```python
from build123d import *

# Parameters (mm, degrees)
SKETCH1_R               = 12.7
BOSS_EXTRUDE1_DEPTH     = 1
CUT_EXTRUDE1_DEPTH      = 18.98832955
CUT_EXTRUDE1_DEPTH_BACK = 18.98832955
SKETCH19_R              = 1
CUT_EXTRUDE2_DEPTH      = 18.98832955
CUT_EXTRUDE2_DEPTH_BACK = 18.98832955
SKETCH20_R              = 7.5
SKETCH21_W              = 65.874202484
SKETCH21_H              = 51.979273979
CUT_EXTRUDE3_DEPTH      = 18.98832955
CUT_EXTRUDE4_DEPTH      = 18.98832955
CUT_EXTRUDE4_DEPTH_BACK = 18.98832955
SKETCH22_R              = 1
SKETCH22_R_2            = 0.25


with BuildPart() as part:
    # Sketch1 → Boss-Extrude1 (new body)
    with BuildSketch(Plane(origin=(0, 0, 0), x_dir=(1, 0, 0), z_dir=(0, 1, 0))):
        with Locations(Location((0, 0, 0), (0, 0, 270))):
            Circle(SKETCH1_R)
    extrude(amount=BOSS_EXTRUDE1_DEPTH)

    # Sketch19 → Cut-Extrude1 (cut, two sides: drawn at the far end of the back side and taken through both)
    with BuildSketch(Plane(origin=(0, 1, 0), x_dir=(1, 0, 0), z_dir=(0, 1, 0)).offset(-CUT_EXTRUDE1_DEPTH_BACK)):
        with Locations(Location((0, 11, 0), (0, 0, 270))):
            Circle(SKETCH19_R)
        with Locations(Location((9.526279442, 5.5, 0), (0, 0, 270))):
            Circle(SKETCH19_R)
        with Locations(Location((9.526279442, -5.5, 0), (0, 0, 270))):
            Circle(SKETCH19_R)
        with Locations(Location((0, -11, 0), (0, 0, 270))):
            Circle(SKETCH19_R)
        with Locations(Location((-9.526279442, -5.5, 0), (0, 0, 270))):
            Circle(SKETCH19_R)
        with Locations(Location((-9.526279442, 5.5, 0), (0, 0, 270))):
            Circle(SKETCH19_R)
    extrude(amount=CUT_EXTRUDE1_DEPTH + CUT_EXTRUDE1_DEPTH_BACK, mode=Mode.SUBTRACT)

    # Sketch20 → Cut-Extrude2 (cut, two sides: drawn at the far end of the back side and taken through both)
    with BuildSketch(Plane(origin=(0, 1, 0), x_dir=(1, 0, 0), z_dir=(0, 1, 0)).offset(-CUT_EXTRUDE2_DEPTH_BACK)):
        with Locations(Location((0, 0, 0), (0, 0, 270))):
            Circle(SKETCH20_R)
    extrude(amount=CUT_EXTRUDE2_DEPTH + CUT_EXTRUDE2_DEPTH_BACK, mode=Mode.SUBTRACT)

    # Sketch21 → Cut-Extrude3 (cut, through all)
    with BuildSketch(Plane.XY):
        with Locations((-3.816154381, 6.321647006)):
            Rectangle(SKETCH21_W, SKETCH21_H)
    extrude(amount=CUT_EXTRUDE3_DEPTH, mode=Mode.SUBTRACT)

    # Sketch22 → Cut-Extrude4 (cut, two sides: drawn at the far end of the back side and taken through both)
    with BuildSketch(Plane(origin=(0, 1, 0), x_dir=(1, 0, 0), z_dir=(0, 1, 0)).offset(-CUT_EXTRUDE4_DEPTH_BACK)):
        with Locations(Location((2.847009496, 10.625184089, 0), (0, 0, 270))):
            Circle(SKETCH22_R)
        with Locations(Location((-5.125, 8.876760389, 0), (0, 0, 270))):
            Circle(SKETCH22_R_2)
    extrude(amount=CUT_EXTRUDE4_DEPTH + CUT_EXTRUDE4_DEPTH_BACK, mode=Mode.SUBTRACT)


solid = part.part
```
For this review, take the finished solid that the model builds, in its own axes (mm). Give positions to 0.01 mm unless a question says otherwise; leave off trailing zeros. Loops run counter-clockwise (first coordinate to the right, second up) from the corner with the lowest first, then second, coordinate; pieces in that order, holes last. Notation, with made-up numbers: M -22,-36 L 33,-36 A24 ccw 33,-25 Z; hole C 86.25,-3.5 d8. An arc over 180 degrees is marked long. One line per item, written item: value. Start each with the question number.
Q1. Add section D-D (y = 0.5). Give the boundary of the cut face in (x, z) (3 decimals).
Q2. For L1, parallel to Z at x = 0, y = 0.5; L2, parallel to X at y = 0.65, z = -11; L3, parallel to X at y = 0.1, z = -11.25, list the stretches that pass through material, from the lowest coordinate up.
Q3. Add section C-C (z = -10.25). Give the boundary of the cut face in (x, y).
Q4. Add section A-A (x = 0). Give the boundary of the cut face in (y, z), and give its area (3 significant figures).
Q5. Add section B-B (z = -2.5). Give the boundary of the cut face in (x, y), and give its area (3 significant figures).
Q6. Draft analysis for pull direction Z (two halves, no side actions). For faces 1 (the face through (10.518, 0.493, -5.63)), 2 (the face through (10.1, 0.5, 0)), 3 (the face through (-0.6, 0.5, -11.8)), 4 (the face through (0.279, 0.493, -12.697)), state which applies: released by +Z, released by -Z, zero draft, split by the parting line, or undercut.
Reply:
1. outline: M -12.7,0 A12.7 ccw 12.7,0 L 7.5,0 A7.5 cw -7.5,0 Z; hole C -9.526,-5.5 d2; hole C -5.125,-8.877 d0.5; hole C 0,-11 d2; hole C 2.847,-10.625 d2; hole C 9.526,-5.5 d2
2. L1: -12.7 to -12, -10 to -7.5
2. L2: -6.35 to -1, 1 to 1.92, 3.77 to 6.35
2. L3: -5.89 to -0.97, 0.97 to 2.07, 3.63 to 5.89
3. outline: M -7.5,0 L -0.66,0 L -0.66,1 L -7.5,1 Z; M 0.66,0 L 1.92,0 L 1.92,1 L 0.66,1 Z; M 3.77,0 L 7.5,0 L 7.5,1 L 3.77,1 Z
4. outline: M 0,-12.7 L 1,-12.7 L 1,-12 L 0,-12 Z; M 0,-10 L 1,-10 L 1,-7.5 L 0,-7.5 Z
4. area: 3.20 mm²
5. outline: M -12.45,0 L -7.07,0 L -7.07,1 L -12.45,1 Z; M 7.07,0 L 12.45,0 L 12.45,1 L 7.07,1 Z
5. area: 10.8 mm²
6. face 1: undercut
6. face 2: released by +Z
6. face 3: undercut
6. face 4: released by -Z
